from build123d import *

# Parameters (mm, degrees)
F0_W      = 84
F0_H      = 59
F1_DEPTH  = 3
F0_W_2    = 90.2
F0_H_2    = 65.2
F2_DEPTH  = 15
F0_W_3    = 96
F0_H_3    = 71
F3_DEPTH  = 22
F5_DEPTH  = 6.5
F6_W      = 29
F6_H      = 12
F7_DEPTH  = 3.2
F8_W      = 29
F8_H      = 12
F9_DEPTH  = 3.2
F10_W     = 8.9470923394
F10_H     = 12
F11_DEPTH = 3.2
F12_W     = 54
F12_H     = 12
F13_DEPTH = 3.2
F14_R     = 1


with BuildPart() as f1:
    # F0 (on Top) → F1 (new body)
    with BuildSketch(Plane.XY):
        Rectangle(F0_W, F0_H)
    extrude(amount=F1_DEPTH)

    # F0 (on Top) → F2 (join)
    with BuildSketch(Plane.XY):
        Rectangle(F0_W_2, F0_H_2)
        Rectangle(F0_W, F0_H, mode=Mode.SUBTRACT)
    extrude(amount=F2_DEPTH)

    # F0 (on Top) → F3 (join)
    with BuildSketch(Plane.XY):
        Rectangle(F0_W_3, F0_H_3)
        Rectangle(F0_W_2, F0_H_2, mode=Mode.SUBTRACT)
    extrude(amount=F3_DEPTH)

    # F4 (on face) → F5 (cut)
    with BuildSketch(Plane.XZ.offset(35.5)):
        Polygon((13.7292444706, 14.0734170091), (13.7292444706, 22), (-13.7292444706, 22), (-13.7292444706, 14.0734170091), (0, 6.1468340183), align=None)
    extrude(amount=-F5_DEPTH, mode=Mode.SUBTRACT)

    # F6 (on face) → F7 (cut)
    with BuildSketch(Plane.YZ.offset(-42)):
        with Locations((0, 9)):
            Rectangle(F6_W, F6_H)
    extrude(amount=-F7_DEPTH, mode=Mode.SUBTRACT)

    # F8 (on face) → F9 (cut)
    with BuildSketch(Plane(origin=(42, 0, 0), x_dir=(0, -1, 0), z_dir=(-1, 0, 0))):
        with Locations((0, 9)):
            Rectangle(F8_W, F8_H)
    extrude(amount=-F9_DEPTH, mode=Mode.SUBTRACT)

    # F10 (on face) → F11 (cut)
    with BuildSketch(Plane(origin=(0, -29.5, 0), x_dir=(-1, 0, 0), z_dir=(0, 1, 0))):
        with Locations((-22.5264538303, 9)):
            Rectangle(F10_W, F10_H)
        with Locations((22.5264538303, 9)):
            Rectangle(F10_W, F10_H)
    extrude(amount=-F11_DEPTH, mode=Mode.SUBTRACT)

    # F12 (on face) → F13 (cut)
    with BuildSketch(Plane.XZ.offset(-29.5)):
        with Locations((0, 9)):
            Rectangle(F12_W, F12_H)
    extrude(amount=-F13_DEPTH, mode=Mode.SUBTRACT)

    # F14
    f14_edges = [f1.edges().sort_by_distance(p)[0] for p in [
        (-30.864622, -35.5, 22),
        (-48, 0, 22),
        (-48, -35.5, 11),
        (48, -35.5, 11),
        (48, 0, 0),
        (0, -35.5, 0),
        (30.864622, -35.5, 22),
        (6.864622, -35.5, 10.110126),
        (-6.864622, -35.5, 10.110126),
        (-13.729244, -35.5, 18.036709),
        (13.729244, -35.5, 18.036709),
        (48, 0, 22),
        (48, 35.5, 11),
        (0, 35.5, 22),
        (0, 35.5, 0),
        (-48, 35.5, 11),
        (-48, 0, 0),
        (0, 32.6, 22),
        (-45.1, 0, 22),
        (45.1, 0, 22),
        (29.414622, -32.6, 22),
        (-29.414622, -32.6, 22),
        (6.864622, -29.5, 10.110126),
        (-6.864622, -29.5, 10.110126),
        (0, -32.5, 6.146834),
    ]]
    fillet(f14_edges, radius=F14_R)


solid = f1.part
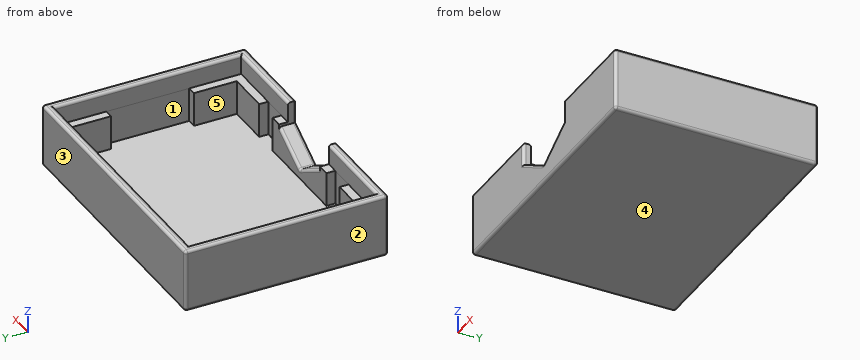
Can you work these out from the model? Positions are in its coordinate system, mm. Face numbers are marked on the shaded views. A direction names the side the tool comes from. Give positions to 0.01 mm unless a question says otherwise; leave off trailing zeros. Write each loop counter-clockwise with the first axis right and the second up, starting at its lowest first coordinate (ties: lowest second). Pieces come first, ordered by that corner, then holes. Notation, with made-up numbers: M 2.5,58.25 L 56.5,58.25 A35 ccw 56.5,95.25 Z; hole C 22,-1.75 d11. An arc over 180 degrees is marked long. Answer in a Markdown table with one row per item. Add a question column.
Item 1: Imagine slicing it at A-A, the plane x = -20. Write out the boundary of the cut face in (y, z).
Item 2: Imagine slicing it at B-B, the plane y = -12.5. Write out the boundary of the cut face in (x, z).
Item 3: On a 3-axis mill with a long thin cutter (end or side, diameter ignored), from which of +Z, -Z, +X, -X, +Y, -Y can I reach the whole of each face in a straight line? I mean the marked faces 4 and 5. Say none if no direction works.
Item 4: For pin 1 Ø10 at (x, y) = (22, -27.5) entering from +Z; pin 2 Ø1 at (x, z) = (-6.5, 13.5) entering from -Y; pin 3 Ø3 at (x, y) = (11.5, 7) entering from +Z, each with a flat end and sliding along its axis, tell me the tip position at first contact or that it passes through.
Item 5: We'd pull the mould along X, two halves only. Please class the marked faces 1, 2 and 3: released by +X, released by -X, zero draft, split by the parting line, or undercut.
Item 6: Please list where these lines run through material, in increasing order: L1, parallel to Y at x = -20, z = 13; L2, parallel to X at y = -31.5, z = 20; L3, parallel to X at y = -4, z = 3.75.
Evaluation:
| question | item | result |
|---|---|---|
| 1 | outline | M -35.5,1 A1 ccw -34.5,0 L 34.5,0 A1 ccw 35.5,1 L 35.5,21 A1 ccw 34.5,22 L 33.6,22 A1 ccw 32.6,21 L 32.6,15 L 32.7,15 L 32.7,3 L -32.7,3 L -32.7,15 L -32.6,15 L -32.6,21 A1 ccw -33.6,22 L -34.5,22 A1 ccw -35.5,21 Z |
| 2 | outline | M -48,1 A1 ccw -47,0 L 47,0 A1 ccw 48,1 L 48,21 A1 ccw 47,22 L 46.1,22 A1 ccw 45.1,21 L 45.1,15 L 45.2,15 L 45.2,3 L -45.2,3 L -45.2,15 L -45.1,15 L -45.1,21 A1 ccw -46.1,22 L -47,22 A1 ccw -48,21 Z |
| 3 | face 4 | -Z, +X, -X, +Y, -Y |
| 3 | face 5 | +Z |
| 4 | pin 1 | stops at z = 15 |
| 4 | pin 2 | stops at y = 32.7 |
| 4 | pin 3 | stops at z = 3 |
| 5 | face 1 | undercut |
| 5 | face 2 | released by -X |
| 5 | face 3 | zero draft |
| 6 | L1 | y = -35.5 to -32.7, 32.7 to 35.5 |
| 6 | L2 | x = -48 to -45.1, 45.1 to 48 |
| 6 | L3 | x = -48 to -45.2, 45.2 to 48 |
